Work out the finished part from the listing and answer in its coordinate system (mm). A direction names the side the tool comes from. Round coordinates to 2 decimals unless told otherwise and drop trailing zeros. Order: outer loops, then holes, each group sorted by start corner. A loop starts at its lowest first (then second) coordinate and runs counter-clockwise, first axis right, second up. Notation, with made-up numbers: (60, 9.5) -> (89, 9.5) arc R20 ccw to (89, 28.5) -> close; hole circle Ø8 at (3.25, 26). An arc over 180 degrees is marked (long way). Use a Markdown table: item, result. Add a question column.
Item 1: Flat-ended cylindrical pins translate along their axes: P1, Ø2, axis at x = -8, z = 1, coming from the +Y side; P2, Ø2, axis at x = 13.02, y = 0, coming from the -Z side. Find the tip coordinate at first contact, or state that the pin passes through.
Item 2: A tool of negligible diameter and unlimited length cuts with its end or side. For faces 4 (the flat face through (-6, 5, 2)), 5 (the flat face through (19.4, -3.2, 2.2)), from which of +Z, -Z, +X, -X, +Y, -Y can it reach the whole face along a straight path? Write none if from no direction.
Item 3: A cutting plane is placed at B-B, the plane x = -10.5. Determine the outline of the cut face in (y, z).
Item 4: For a pull along X with two mould halves and no side action, classify faces 1 (the cylindrical face through (14.7, 0.5, 2.2)), 2 (the flat face through (47.797, 8.043, 2.218)), 3 (the flat face through (2, -5, 2)) as +X half, -X half, draft (parallel to the pull), parting line (faces both ways), or undercut.
Item 5: A cutting plane is placed at A-A, the plane z = 3.2. Give the number of separate pieces and of enclosed holes in the cut face, plus the area to 3 significant figures.
Item 6: Find the intervals of material crossed by L1, parallel to X at y = 1.5, z = 1.35; L2, parallel to Y at x = -3, z = 4.05; L3, parallel to Y at x = 42, z = 2.2, in increasing order. Write a range as [from, to].
from build123d import *

# Parameters (mm, degrees)
SKETCH1_R           = 5
SKETCH1_R_2         = 1.75
BOSS_EXTRUDE1_DEPTH = 4.5
BOSS_EXTRUDE2_START = -4.5
BOSS_EXTRUDE2_DEPTH = 4.5


with BuildPart() as part:
    # Sketch1 → Boss-Extrude1 (new body)
    # profile 1 of 3: a face of its own
    with BuildSketch(Plane.XY):
        with Locations((-13.023088496, 0)):
            Circle(SKETCH1_R)
        with Locations((-13.023088496, 0)):
            Circle(SKETCH1_R_2, mode=Mode.SUBTRACT)
    # profile 2 of 3: a face of its own
    with BuildSketch(Plane.XY):
        with Locations((13.023088496, 0)):
            Circle(SKETCH1_R)
        with Locations((13.023088496, 0)):
            Circle(SKETCH1_R_2, mode=Mode.SUBTRACT)
    # profile 3 of 3: a face of its own
    with BuildSketch(Plane.XY):
        with BuildLine():
            Line((-13.023088477, -5), (13.023088496, -5))
            ThreePointArc((13.023088496, -5), (8.023088496, 0), (13.023088496, 5))
            Line((13.023088496, 5), (-13.02308848, 5))
            ThreePointArc((-13.02308848, 5), (-9.487554585, 3.5355339), (-8.023088496, 0))
            ThreePointArc((-8.023088496, 0), (-9.487554584, -3.535533899), (-13.023088477, -5))
        make_face()
    extrude(amount=BOSS_EXTRUDE1_DEPTH)

    # Sketch2 → Boss-Extrude2 (add)
    with BuildSketch(Plane.XY.offset(4.5).offset(BOSS_EXTRUDE2_START)):
        with BuildLine():
            Line((48.387077696, 12.87), (51.203884398, 10.03))
            Line((51.203884398, 10.03), (44.293088496, 6))
            add(Edge.make_bspline(
                [(44.293088496, 6), (32.169239244, 6.157348305), (22.633088496, -1.48)],
                knots=[0, 0, 0, 1, 1, 1], degree=2))
            Line((22.633088496, -1.48), (16.013088496, -5))
            Line((16.013088496, -5), (13.023088496, -5))
            ThreePointArc((13.023088496, -5), (18.023088496, 0), (13.023088496, 5))
            Line((13.023088496, 5), (0, 5))
            add(Edge.make_bspline(
                [(0, 5), (23.957075796, 10.418061583), (48.387077696, 12.87)],
                knots=[0, 0, 0, 1, 1, 1], degree=2))
        make_face()
    extrude(amount=BOSS_EXTRUDE2_DEPTH)


solid = part.part
Reported:
| question | item | result |
|---|---|---|
| 1 | P1 | y = 5 |
| 1 | P2 | through |
| 2 | face 4 | +Z, -Z, -X, +Y |
| 2 | face 5 | +Z, -Z, +X, -Y |
| 3 | outline | (-5, 0) -> (5, 0) -> (5, 4.5) -> (-5, 4.5) -> close |
| 4 | face 1 | undercut |
| 4 | face 2 | +X half |
| 4 | face 3 | draft |
| 5 | separate pieces | 1 |
| 5 | enclosed holes | 2 |
| 5 | area | 605 mm² |
| 6 | L1 | [-17.79, -13.92], [-12.12, 12.12], [13.92, 26.95] |
| 6 | L2 | [-5, 5] |
| 6 | L3 | [5.96, 12.18] |
